```python
from build123d import *

# Parameters (mm, degrees)
F0_R      = 2.25
F0_R_2    = 1
F1_DEPTH  = 4
F2_W      = 12
F2_H      = 12
F2_R      = 2.25
F3_DEPTH  = 6
F4_W      = 8
F4_H      = 8
F4_R      = 2.25
F5_DEPTH  = 2
F6_R      = 4
F6_R_2    = 2.25
F7_DEPTH  = 5
F8_R      = 2.5
F8_R_2    = 1
F9_DEPTH  = 4
F11_DEPTH = 4.001


# Not quite as in the source:
# - a feature names something its author has since deleted; it is built from what else it names


with BuildPart() as f1:
    # F0 (on Top) → F1 (new body)
    with BuildSketch(Plane.XY):
        Polygon((-43.4, 46), (-55.4, 46), (-55.4, -46), (-43.4, -46), (-43.4, -34), (-0.4, -34), (-0.4, -46), (11.6, -46), (11.6, -34), (30.1, -34), (30.1, 34), (11.6, 34), (11.6, 46), (-0.4, 46), (-0.4, 34), (-43.4, 34), align=None)
        with Locations((-49.4, -40)):
            Circle(F0_R, mode=Mode.SUBTRACT)
        with Locations((-30, -13)):
            Circle(F0_R_2, mode=Mode.SUBTRACT)
        with Locations((5.6, -40)):
            Circle(F0_R, mode=Mode.SUBTRACT)
        with Locations((-49.4, 40)):
            Circle(F0_R, mode=Mode.SUBTRACT)
        with Locations((25.1, 10.5)):
            Circle(F0_R_2, mode=Mode.SUBTRACT)
        with Locations((5.6, 40)):
            Circle(F0_R, mode=Mode.SUBTRACT)
    extrude(amount=F1_DEPTH)

    # F2 (on face) → F3 (join)
    with BuildSketch(Plane.XY.offset(4)):
        with Locations((-49.4, -40)):
            Rectangle(F2_W, F2_H)
        with Locations((-49.4, -40)):
            Circle(F2_R, mode=Mode.SUBTRACT)
        with Locations((-49.4, 40)):
            Rectangle(F2_W, F2_H)
        with Locations((-49.4, 40)):
            Circle(F2_R, mode=Mode.SUBTRACT)
        with Locations((5.6, 40)):
            Rectangle(F2_W, F2_H)
        with Locations((5.6, 40)):
            Circle(F2_R, mode=Mode.SUBTRACT)
        with Locations((5.6, -40)):
            Rectangle(F2_W, F2_H)
        with Locations((5.6, -40)):
            Circle(F2_R, mode=Mode.SUBTRACT)
    extrude(amount=F3_DEPTH)

    # F4 (on face) → F5 (cut)
    with BuildSketch(Plane.XY.offset(10)):
        with Locations((-49.4, 40)):
            Rectangle(F4_W, F4_H)
        with Locations((-49.4, 40)):
            Circle(F4_R, mode=Mode.SUBTRACT)
        with Locations((5.6, 40)):
            Rectangle(F4_W, F4_H)
        with Locations((5.6, 40)):
            Circle(F4_R, mode=Mode.SUBTRACT)
        with Locations((5.6, -40)):
            Rectangle(F4_W, F4_H)
        with Locations((5.6, -40)):
            Circle(F4_R, mode=Mode.SUBTRACT)
        with Locations((-49.4, -40)):
            Rectangle(F4_W, F4_H)
        with Locations((-49.4, -40)):
            Circle(F4_R, mode=Mode.SUBTRACT)
    extrude(amount=-F5_DEPTH, mode=Mode.SUBTRACT)

    # F6 (on face) → F7 (cut)
    with BuildSketch(Plane(origin=(0, 0, 0), x_dir=(1, 0, 0), z_dir=(0, 0, -1))):
        with Locations((-49.4, 40)):
            Circle(F6_R)
        with Locations((-49.4, 40)):
            Circle(F6_R_2, mode=Mode.SUBTRACT)
        with Locations((5.6, 40)):
            Circle(F6_R)
        with Locations((5.6, 40)):
            Circle(F6_R_2, mode=Mode.SUBTRACT)
        with Locations((5.6, -40)):
            Circle(F6_R)
        with Locations((5.6, -40)):
            Circle(F6_R_2, mode=Mode.SUBTRACT)
        with Locations((-49.4, -40)):
            Circle(F6_R)
        with Locations((-49.4, -40)):
            Circle(F6_R_2, mode=Mode.SUBTRACT)
    extrude(amount=-F7_DEPTH, mode=Mode.SUBTRACT)

    # F8 (on face) → F9 (join)
    with BuildSketch(Plane.XY.offset(4)):
        with Locations((-30, -13)):
            Circle(F8_R)
        with Locations((-30, -13)):
            Circle(F8_R_2, mode=Mode.SUBTRACT)
        with Locations((25.1, 10.5)):
            Circle(F8_R)
        with Locations((25.1, 10.5)):
            Circle(F8_R_2, mode=Mode.SUBTRACT)
    extrude(amount=F9_DEPTH)

    # F10 (on face) → F11 (cut, through all)
    with BuildSketch(Plane.XY.offset(4)):
        with BuildLine():
            ThreePointArc((-49.4, 28.25), (-47.8090097423, 27.5909902577), (-47.15, 26))
            ThreePointArc((-47.15, 26), (-47.8090097423, 24.4090097423), (-49.4, 23.75))
            Line((-49.4, 23.75), (24.1, 23.75))
            ThreePointArc((24.1, 23.75), (21.85, 26), (24.1, 28.25))
            Line((24.1, 28.25), (-49.4, 28.25))
        make_face()
        with BuildLine():
            ThreePointArc((-49.4, 23.75), (-47.8090097423, 24.4090097423), (-47.15, 26))
            ThreePointArc((-47.15, 26), (-47.8090097423, 27.5909902577), (-49.4, 28.25))
            ThreePointArc((-49.4, 28.25), (-51.65, 26), (-49.4, 23.75))
        make_face()
        with BuildLine():
            Line((-47.15, -26), (-47.15, 18))
            ThreePointArc((-47.15, 18), (-49.4, 15.75), (-51.65, 18))
            Line((-51.65, 18), (-51.65, -26))
            ThreePointArc((-51.65, -26), (-49.4, -23.75), (-47.15, -26))
        make_face()
        with BuildLine():
            ThreePointArc((-51.65, 18), (-49.4, 15.75), (-47.15, 18))
            ThreePointArc((-47.15, 18), (-49.4, 20.25), (-51.65, 18))
        make_face()
        with BuildLine():
            ThreePointArc((-40.606821277, 16.1010312258), (-38.3166828427, 16.0279645194), (-37.15, 18))
            ThreePointArc((-37.15, 18), (-37.4279645194, 19.0833171573), (-38.193178723, 19.8989687742))
            ThreePointArc((-38.193178723, 19.8989687742), (-41.2989687742, 19.206821277), (-40.606821277, 16.1010312258))
        make_face()
        with BuildLine():
            ThreePointArc((-51.65, -26), (-49.4, -28.25), (-47.15, -26))
            ThreePointArc((-47.15, -26), (-49.4, -23.75), (-51.65, -26))
        make_face()
        with BuildLine():
            ThreePointArc((-39.4, -28.25), (-37.8090097423, -27.5909902577), (-37.15, -26))
            ThreePointArc((-37.15, -26), (-37.8090097423, -24.4090097423), (-39.4, -23.75))
            ThreePointArc((-39.4, -23.75), (-41.65, -26), (-39.4, -28.25))
        make_face()
        with BuildLine():
            ThreePointArc((-39.4, -23.75), (-37.8090097423, -24.4090097423), (-37.15, -26))
            ThreePointArc((-37.15, -26), (-37.8090097423, -27.5909902577), (-39.4, -28.25))
            Line((-39.4, -28.25), (14.1, -28.25))
            ThreePointArc((14.1, -28.25), (11.85, -26), (14.1, -23.75))
            Line((14.1, -23.75), (-39.4, -23.75))
        make_face()
        with BuildLine():
            ThreePointArc((16.35, -26), (15.6909902577, -24.4090097423), (14.1, -23.75))
            ThreePointArc((14.1, -23.75), (11.85, -26), (14.1, -28.25))
            ThreePointArc((14.1, -28.25), (15.6909902577, -27.5909902577), (16.35, -26))
        make_face()
        with BuildLine():
            ThreePointArc((21.85, -26), (24.1, -28.25), (26.35, -26))
            ThreePointArc((26.35, -26), (24.1, -23.75), (21.85, -26))
        make_face()
        with BuildLine():
            ThreePointArc((16.35, -16), (16.0720354806, -14.9166828427), (15.306821277, -14.1010312258))
            ThreePointArc((15.306821277, -14.1010312258), (12.2010312258, -14.793178723), (12.893178723, -17.8989687742))
            ThreePointArc((12.893178723, -17.8989687742), (15.1833171573, -17.9720354806), (16.35, -16))
        make_face()
        with BuildLine():
            ThreePointArc((-38.193178723, 19.8989687742), (-37.4279645194, 19.0833171573), (-37.15, 18))
            ThreePointArc((-37.15, 18), (-38.3166828427, 16.0279645194), (-40.606821277, 16.1010312258))
            Line((-40.606821277, 16.1010312258), (12.893178723, -17.8989687742))
            ThreePointArc((12.893178723, -17.8989687742), (12.2010312258, -14.793178723), (15.306821277, -14.1010312258))
            Line((15.306821277, -14.1010312258), (-38.193178723, 19.8989687742))
        make_face()
        with BuildLine():
            ThreePointArc((21.85, -26), (24.1, -23.75), (26.35, -26))
            Line((26.35, -26), (26.35, 2.5))
            ThreePointArc((26.35, 2.5), (24.1, 0.25), (21.85, 2.5))
            Line((21.85, 2.5), (21.85, -26))
        make_face()
        with BuildLine():
            ThreePointArc((21.85, 2.5), (24.1, 0.25), (26.35, 2.5))
            ThreePointArc((26.35, 2.5), (24.1, 4.75), (21.85, 2.5))
        make_face()
        with BuildLine():
            ThreePointArc((26.35, 26), (25.6909902577, 27.5909902577), (24.1, 28.25))
            ThreePointArc((24.1, 28.25), (21.85, 26), (24.1, 23.75))
            ThreePointArc((24.1, 23.75), (25.6909902577, 24.4090097423), (26.35, 26))
        make_face()
    extrude(amount=-F11_DEPTH, mode=Mode.SUBTRACT)


solid = f1.part
```
The listing builds one solid part. Answer for the finished solid, in the listing's coordinates (mm). A direction names the side the tool comes from. Round coordinates to 2 decimals unless told otherwise and drop trailing zeros.
1) A cutting plane is placed at A-A on z = 6.75. Give the number of separate pieces and of enclosed holes in the cut face, plus the area to 3 significant figures.
Outcome:
separate pieces: 6
enclosed holes: 6
area: 545 mm2
2) For a pull along X with two mould halves and no side action, classify faces 6 (the face through (6, -34, 7)), 7 (the face through (-43.4, -40, 5)) as released by +X, released by -X, zero draft, split by the parting line, or undercut.
Outcome:
face 6: zero draft
face 7: undercut
3) Consider line 1 (Y direction, x = 5.6, z = 5.85); line 2 (Y direction, x = 5.6, z = 2.6); line 3 (X direction, y = -40, z = 6.8). Determine where each line is inside the solid, lowest interval first.
Outcome:
line 1: y = -46 to -42.25, -37.75 to -34, 34 to 37.75, 42.25 to 46
line 2: y = -46 to -44, -36 to -28.25, -23.75 to -13.26, -7.93 to 23.75, 28.25 to 36, 44 to 46
line 3: x = -55.4 to -51.65, -47.15 to -43.4, -0.4 to 3.35, 7.85 to 11.6
4) For faces 1 (the face through (5.079, 36.034, 2.465)), 2 (the face through (-49, -46, 5)), 3 (the face through (1.6, -40, 9)), 4 (the face through (-14.23, -0.66, 2.03)), 5 (the face through (-22, 34, 2)), determine the directions among +Z, -Z, +X, -X, +Y, -Y from which every point of the face is accessible in a straight line to the end or side of a thin tool.
Outcome:
face 1: -Z
face 2: +Z, -Z, +X, -X, -Y
face 3: +Z
face 4: +Z, -Z
face 5: +Z, -Z, +Y
5) Given P1, Ø2.5, axis at x = 25.1, y = 10.5, coming from the +Z side; P2, Ø5, axis at x = 21.5, z = 8.5, coming from the -Y side; P3, Ø0.6, axis at y = -40, z = 9.5, coming from the +X side, each flat-ended and moving along its own axis, determine where each tip first touches the part or whether it passes through.
Outcome:
P1: stops at z = 8
P2: stops at y = 8.28
P3: stops at x = 11.6
